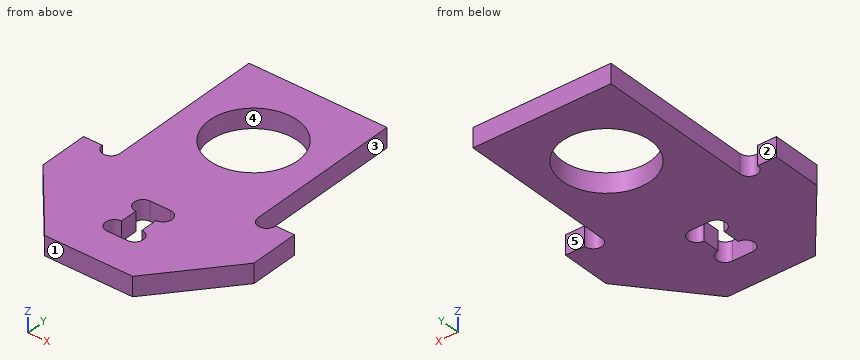
from build123d import *

# Parameters (mm, degrees)
SKETCH_1_R      = 5
EXTRUDE_1_DEPTH = 2.2


with BuildPart() as part:
    # 草图1 → 凸台-拉伸1 (new body)
    with BuildSketch(Plane.XY):
        with BuildLine():
            Line((-7.85, 9), (-7.85, -9))
            ThreePointArc((-7.85, -9), (-8.855, -10.005), (-9.86, -9))
            Line((-9.86, -9), (-12, -9))
            Line((-12, -9), (-12, -14.657724852))
            Line((-12, -14.657724852), (-5, -23))
            Line((-5, -23), (5, -23))
            Line((5, -23), (12, -14.657724852))
            Line((12, -14.657724852), (12, -9))
            Line((12, -9), (9.86, -9))
            ThreePointArc((9.86, -9), (8.855, -10.005), (7.85, -9))
            Line((7.85, -9), (7.85, 9))
            Line((7.85, 9), (-7.85, 9))
        make_face()
        with BuildLine():
            ThreePointArc((2.155, -17.995), (1.860642315, -18.705642315), (1.15, -19))
            Line((1.15, -19), (-1.15, -19))
            ThreePointArc((-1.15, -19), (-2.155, -17.995), (-1.15, -16.99))
            Line((-1.15, -16.99), (-1.15, -15.01))
            ThreePointArc((-1.15, -15.01), (-2.155, -14.005), (-1.15, -13))
            Line((-1.15, -13), (1.15, -13))
            ThreePointArc((1.15, -13), (1.860642315, -13.294357685), (2.155, -14.005))
            ThreePointArc((2.155, -14.005), (1.860642315, -14.715642315), (1.15, -15.01))
            Line((1.15, -15.01), (1.15, -16.99))
            ThreePointArc((1.15, -16.99), (1.860642315, -17.284357685), (2.155, -17.995))
        make_face(mode=Mode.SUBTRACT)
        Circle(SKETCH_1_R, mode=Mode.SUBTRACT)
    extrude(amount=EXTRUDE_1_DEPTH)


solid = part.part
Input: part model. Units: mm. Frame: model coordinates. Face numbers are marked on the shaded views. A direction names the side the tool comes from. Coordinates: 2 decimals unless noted, no trailing zeros. Loops run counter-clockwise (first coordinate to the right, second up) from the corner with the lowest first, then second, coordinate; pieces in that order, holes last.
Q1. Set-up query: the marked faces 1 and 2. Return all of +Z, -Z, +X, -X, +Y, -Y with unobstructed straight access to the full face (end or side cutting, diameter ignored); none if empty.
Q2. Material intervals for line 1 (Y direction, x = 0, z = 1.65); line 2 (X direction, y = 7, z = 0.3); line 3 (Y direction, x = -3.75, z = 0.4), sorted ascending.
Q3. Cut plane A-A (x = 0). Output: boundary loops of the cut face in (y, z).
Q4. Cut plane B-B (y = 0). Output: boundary loops of the cut face in (x, z), then the cut area to 3 significant figures.
Q5. Cut plane D-D (x = 3.5). Output: boundary loops of the cut face in (y, z), then the cut area to 3 significant figures.
Q6. Cut plane C-C (z = 1.8). Output: boundary loops of the cut face in (x, y) (3 decimals).
Q7. Contact query for flat-ended pins moving along their axis: pin 1 (6 mm diameter, centred on x = 0, y = 0, fed in from -Z); pin 2 (0.6 mm diameter, centred on x = 11, z = 0.5, fed in from +Y); pin 3 (1 mm diameter, centred on y = -15.5, z = 1, fed in from -X); pin 4 (1 mm diameter, centred on y = -15.5, z = 1.5, fed in from +X). Output: stop coordinate, or through.
Q8. Draft query along Y for the marked faces 3, 4 and 5. Return one class per face: +Y half, -Y half, draft (parallel to the pull), parting line (faces both ways), or undercut.
Working result:
1. face 1: +Z, -Z, +X, -X, -Y
1. face 2: +Z, -Z, -X, +Y
2. line 1: y = -23 to -19, -13 to -5, 5 to 9
2. line 2: x = -7.85 to 7.85
2. line 3: y = -23 to -3.31, 3.31 to 9
3. outline: (-23, 0) - (-19, 0) - (-19, 2.2) - (-23, 2.2) - close; (-13, 0) - (-5, 0) - (-5, 2.2) - (-13, 2.2) - close; (5, 0) - (9, 0) - (9, 2.2) - (5, 2.2) - close
4. outline: (-7.85, 0) - (-5, 0) - (-5, 2.2) - (-7.85, 2.2) - close; (5, 0) - (7.85, 0) - (7.85, 2.2) - (5, 2.2) - close
4. area: 12.5 mm2
5. outline: (-23, 0) - (-3.57, 0) - (-3.57, 2.2) - (-23, 2.2) - close; (3.57, 0) - (9, 0) - (9, 2.2) - (3.57, 2.2) - close
5. area: 54.7 mm2
6. outline: (-12, -14.658) - (-5, -23) - (5, -23) - (12, -14.658) - (12, -9) - (9.86, -9) arc R1.005 cw to (7.85, -9) - (7.85, 9) - (-7.85, 9) - (-7.85, -9) arc R1.005 cw to (-9.86, -9) - (-12, -9) - close; hole circle Ø10 at (0, 0); hole (-1.15, -19) - (1.15, -19) arc R1.005 ccw to (1.15, -16.99) - (1.15, -15.01) arc R1.005 ccw to (1.15, -13) - (-1.15, -13) arc R1.005 ccw to (-1.15, -15.01) - (-1.15, -16.99) arc R1.005 ccw to start
7. pin 1: passes through
7. pin 2: stops at y = -9
7. pin 3: stops at x = -11.71
7. pin 4: stops at x = 11.71
8. face 3: draft
8. face 4: undercut
8. face 5: +Y half
